```python
from build123d import *

# Parameters (mm, degrees)
F0_R     = 27.5
F1_DEPTH = 55
F2_R     = 27.5
F2_R_2   = 21
F3_DEPTH = 50
F5_D     = 35.2


with BuildPart() as f1:
    # F0 (on Front) → F1 (new body)
    with BuildSketch(Plane.XZ):
        Circle(F0_R)
    extrude(amount=-F1_DEPTH)

    # F2 (on face) → F3 (cut)
    with BuildSketch(Plane(origin=(0, 55, 0), x_dir=(-1, 0, 0), z_dir=(0, 1, 0))):
        Circle(F2_R)
        Circle(F2_R_2, mode=Mode.SUBTRACT)
    extrude(amount=-F3_DEPTH, mode=Mode.SUBTRACT)

    # F5 (through all)
    with Locations(Plane.XZ):
        with Locations((0, 0)):
            Hole(F5_D / 2)


solid = f1.part
```
The model under review builds one solid part; all positions refer to its coordinate system, in mm. A direction names the side the tool comes from. Coordinates: 2 decimals unless noted, no trailing zeros. Write each loop counter-clockwise with the first axis right and the second up, starting at its lowest first coordinate (ties: lowest second). Pieces come first, ordered by that corner, then holes. Notation, with made-up numbers: (63.25, -14) -> (69.25, -14) arc R31 ccw to (69.25, 21) -> close; hole circle Ø2 at (43.5, 79.5). An arc over 180 degrees is marked (long way). One line per item, written item: value. Start each with the question number.
Q1. For faces 4 (the face through (0, 0, -18)), 5 (the face through (-20.03, 30.35, 6.31)), list the 3-axis set-ups (+Z, -Z, +X, -X, +Y, -Y) from which the entire face can be reached by the end or side of a thin tool; tool diameter is ignored.
Q2. Add section D-D, the plane y = 35. Give the boundary of the cut face in (x, z), then the cut area to 3 significant figures.
Q3. To check wall thickness, follow probe 1 along Z at (x, y) = (-0.5, 11); probe 2 along Z at (x, y) = (-10, 15.5); probe 3 along Y at (x, z) = (21, 13). State the ranges of each line that lie inside material, in increasing order.
Q4. Add section B-B, the plane x = 0. Give the boundary of the cut face in (y, z), then the cut area to 3 significant figures.
Q5. Add section C-C, the plane x = -20. Give the boundary of the cut face in (y, z).
Q6. Add section A-A, the plane z = 0. Give the boundary of the cut face in (x, y).
Q7. Clearance check with flat-ended pins moving along their axes: P1, Ø5, axis at y = 39, z = -5, coming from the +X side; P2, Ø1, axis at x = -12, y = 19, coming from the -Z side; P3, Ø3, axis at y = 47, z = 18.5, coming from the -X side. State where each tip first meets the part, or that it passes through.
Q8. The part is to be moulded in two halves that separate along X. For faces 1 (the face through (6.24, 5, -20.24)), 2 (the face through (-5.961, 2.465, -26.846)), 3 (the face through (-16.787, 27.885, 5.287)), say which applies: +X half, -X half, draft (parallel to the pull), parting line (faces both ways), or undercut.
Response:
1. face 4: +Z, -Z, +X, -X, -Y
1. face 5: +Y
2. outline: circle Ø42 at (0, 0); hole circle Ø35.2 at (0, 0)
2. area: 412 mm²
3. probe 1: -20.99 to -17.59, 17.59 to 20.99
3. probe 2: -18.47 to -14.48, 14.48 to 18.47
3. probe 3: 0 to 5
4. outline: (0, -27.5) -> (5, -27.5) -> (5, -21) -> (55, -21) -> (55, -17.6) -> (0, -17.6) -> close; (0, 17.6) -> (55, 17.6) -> (55, 21) -> (5, 21) -> (5, 27.5) -> (0, 27.5) -> close
4. area: 439 mm²
5. outline: (0, -18.87) -> (5, -18.87) -> (5, -6.4) -> (55, -6.4) -> (55, 6.4) -> (5, 6.4) -> (5, 18.87) -> (0, 18.87) -> close
6. outline: (-27.5, 0) -> (-17.6, 0) -> (-17.6, 55) -> (-21, 55) -> (-21, 5) -> (-27.5, 5) -> close; (17.6, 0) -> (27.5, 0) -> (27.5, 5) -> (21, 5) -> (21, 55) -> (17.6, 55) -> close
7. P1: x = 20.85
7. P2: z = -17.57
7. P3: x = -12.33
8. face 1: draft
8. face 2: parting line
8. face 3: undercut
